Part model, mm, in its own coordinate system. Face numbers are marked on the shaded views. Coordinates: 2 decimals unless noted, no trailing zeros. Loops run counter-clockwise (first coordinate to the right, second up) from the corner with the lowest first, then second, coordinate; pieces in that order, holes last. Notation, with made-up numbers: (50, -16.5) -> (57, -16.5) arc R30 ccw to (57, 17.5) -> close; hole circle Ø1 at (38.5, -20.75). An arc over 180 degrees is marked (long way). One line per question, with ' | ' between items. Start each with the question number.
1) Drop flat-ended pins along their axis: pin 1 (2.5 mm diameter, centred on x = -143.5, z = 9, fed in from -Y); pin 2 (1.5 mm diameter, centred on x = -511, z = 159.5, fed in from +Y). Give the stop position or say it passes through.
2) Two-plate mould, pull along X, no slides. Class the marked faces 1 and 2: released by +X, released by -X, zero draft, split by the parting line, or undercut.
3) Probe L1, parallel to Z at x = -12, y = 10.5; L2, parallel to Z at x = -132, y = 31.5; L3, parallel to X at y = 20, z = 376. List the from-to ranges inside material, lowest first. Write a range as from..to.
4) Cut at A-A (x = -461). List the corners of the cut face in (y, z).
5) Cut at B-B (z = 112.5). List the corners of the cut face in (x, y), plus the area to 3 significant figures.
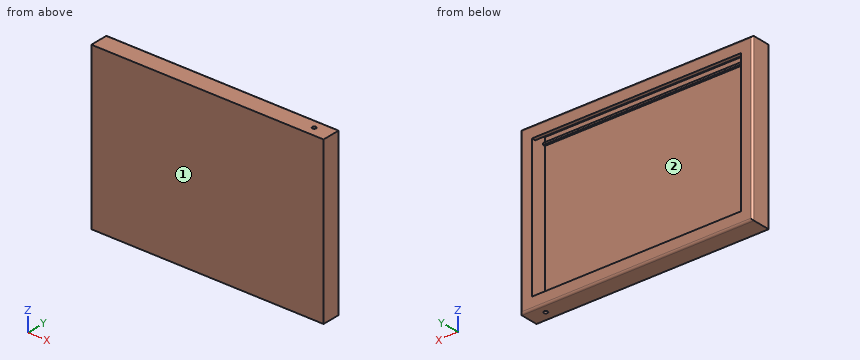
from build123d import *

# Parameters (mm, degrees)
SKETCH_1_W          = 600
SKETCH_1_H          = 420
EXTRUDE_1_DEPTH     = 50
SKETCH_2_W          = 540
SKETCH_2_H          = 360
CUT_EXTRUDE_1_DEPTH = 40
SKETCH_3_W          = 540
SKETCH_3_H          = 30
CUT_EXTRUDE_2_DEPTH = 20
SKETCH_4_W          = 540
SKETCH_4_H          = 30
CUT_EXTRUDE_3_DEPTH = 20
SKETCH_6_W          = 540
SKETCH_6_H          = 5
EXTRUDE_3_DEPTH     = 40
SKETCH_7_W          = 540
SKETCH_7_H          = 5
EXTRUDE_4_DEPTH     = 40
SKETCH_8_W          = 540
SKETCH_8_H          = 30
CUT_EXTRUDE_4_DEPTH = 20
SKETCH_9_W          = 540
SKETCH_9_H          = 30
CUT_EXTRUDE_5_DEPTH = 20
SKETCH_11_W         = 540
SKETCH_11_H         = 5
EXTRUDE_6_DEPTH     = 10
SKETCH_12_R         = 5
CUT_EXTRUDE_6_DEPTH = 711.815967718
FILLET_1_R          = 5


with BuildPart() as part:
    # 스케치1 → 보스-돌출1 (new body)
    with BuildSketch(Plane(origin=(0, 0, 0), x_dir=(1, 0, 0), z_dir=(0, 1, 0))):
        with Locations((-271.278688525, -192)):
            Rectangle(SKETCH_1_W, SKETCH_1_H)
    extrude(amount=EXTRUDE_1_DEPTH)

    # 스케치2 → 컷-돌출1 (cut)
    with BuildSketch(Plane(origin=(0, 50, 0), x_dir=(1, 0, 0), z_dir=(0, 1, 0))):
        with Locations((-271.278688525, -192)):
            Rectangle(SKETCH_2_W, SKETCH_2_H)
    extrude(amount=-CUT_EXTRUDE_1_DEPTH, mode=Mode.SUBTRACT)

    # 스케치3 → 컷-돌출2 (cut)
    with BuildSketch(Plane.XY.offset(12)):
        with Locations((-271.278688525, 25)):
            Rectangle(SKETCH_3_W, SKETCH_3_H)
    extrude(amount=-CUT_EXTRUDE_2_DEPTH, mode=Mode.SUBTRACT)

    # 스케치4 → 컷-돌출3 (cut)
    with BuildSketch(Plane(origin=(0, 0, 372), x_dir=(-1, 0, 0), z_dir=(0, 0, -1))):
        with Locations((271.278688525, 25)):
            Rectangle(SKETCH_4_W, SKETCH_4_H)
    extrude(amount=-CUT_EXTRUDE_3_DEPTH, mode=Mode.SUBTRACT)

    # 스케치6 → 보스-돌출3 (add)
    with BuildSketch(Plane(origin=(0, 50, 0), x_dir=(1, 0, 0), z_dir=(0, 1, 0))):
        with Locations((-271.278688525, -9.5)):
            Rectangle(SKETCH_6_W, SKETCH_6_H)
    extrude(amount=-EXTRUDE_3_DEPTH)

    # 스케치7 → 보스-돌출4 (add)
    with BuildSketch(Plane(origin=(0, 50, 0), x_dir=(1, 0, 0), z_dir=(0, 1, 0))):
        with Locations((-271.278688525, -374.5)):
            Rectangle(SKETCH_7_W, SKETCH_7_H)
    extrude(amount=-EXTRUDE_4_DEPTH)

    # 스케치8 → 컷-돌출4 (cut)
    with BuildSketch(Plane(origin=(0, 0, 372), x_dir=(-1, 0, 0), z_dir=(0, 0, -1))):
        with Locations((271.278688525, 30)):
            Rectangle(SKETCH_8_W, SKETCH_8_H)
    extrude(amount=-CUT_EXTRUDE_4_DEPTH, mode=Mode.SUBTRACT)

    # 스케치9 → 컷-돌출5 (cut)
    with BuildSketch(Plane.XY.offset(12)):
        with Locations((-271.278688525, 30)):
            Rectangle(SKETCH_9_W, SKETCH_9_H)
    extrude(amount=-CUT_EXTRUDE_5_DEPTH, mode=Mode.SUBTRACT)

    # 스케치11 → 보스-돌출6 (add)
    with BuildSketch(Plane(origin=(0, 50, 0), x_dir=(1, 0, 0), z_dir=(0, 1, 0))):
        with Locations((-271.278688525, -9.5)):
            Rectangle(SKETCH_11_W, SKETCH_11_H)
        with Locations((-271.278688525, -374.5)):
            Rectangle(SKETCH_11_W, SKETCH_11_H)
    extrude(amount=-EXTRUDE_6_DEPTH)

    # 스케치12 → 컷-돌출6 (cut, through all)
    with BuildSketch(Plane.XY.offset(402)):
        with Locations((-16.278688525, 25)):
            Circle(SKETCH_12_R)
    extrude(amount=-CUT_EXTRUDE_6_DEPTH, mode=Mode.SUBTRACT)

    # 필렛1
    fillet_1_edges = [part.edges().sort_by_distance(p)[0] for p in [
        (28.721311475, 50, 192),
        (-271.278688525, 50, -18),
        (-571.278688525, 50, 192),
        (-271.278688525, 50, 402),
    ]]
    fillet(fillet_1_edges, radius=FILLET_1_R)


solid = part.part
Reported:
1) pin 1: stops at y = 0 | pin 2: stops at y = 10
2) face 1: zero draft | face 2: undercut
3) L1: z = -18..-8, 7..12, 372..377, 392..402 | L2: z = -18..-8, 392..402 | L3: x = -571.28..-541.28, -1.28..28.72
4) outline: (0, -18) -> (45, -18) arc R5 ccw to (50, -13) -> (50, 12) -> (40, 12) -> (40, 7) -> (45, 7) -> (45, -8) -> (10, -8) -> (10, 7) -> (15, 7) -> (15, 12) -> (10, 12) -> (10, 372) -> (15, 372) -> (15, 377) -> (10, 377) -> (10, 392) -> (45, 392) -> (45, 377) -> (40, 377) -> (40, 372) -> (50, 372) -> (50, 397) arc R5 ccw to (45, 402) -> (0, 402) -> close
5) outline: (-571.28, 0) -> (28.72, 0) -> (28.72, 45) arc R5 ccw to (23.72, 50) -> (-1.28, 50) -> (-1.28, 10) -> (-541.28, 10) -> (-541.28, 50) -> (-566.28, 50) arc R5 ccw to (-571.28, 45) -> close | area: 8,390 mm²
